Autodesk Inventor part; units mm, degrees
ref_plane "YZ Plane" through (0, 0, 0) normal (1, 0, 0) x (0, 1, 0)
ref_plane "XZ Plane" through (0, 0, 0) normal (0, 1, 0) x (-1, 0, 0)
ref_plane "XY Plane" through (0, 0, 0) normal (0, 0, 1) x (1, 0, 0)
sketch "Skizze1" plane through (0, 0, 0) normal (0, 0, 1) x (1, 0, 0)
  circle A0 centre (0, 0) radius 9.75
  dimension "d0" = 19.5
extrude "Extrusion1" add sketch "Skizze1" along normal blind 830
sketch "Skizze4" plane through (0, 0, 830) normal (0, 0, 1) x (1, 0, 0)
  arc A0 (0, -25) -> (0, 25) centre (0, 0) ccw
  line L0 (0, 0) -> (0, -25) construction
  line L1 (0, 0) -> (0, 27.5151) construction
  line L2 (0, 25) -> (-100, 25)
  line L3 (-100, 25) -> (-100, -25)
  line L4 (-100, -25) -> (0, -25)
  point P0 (0, 25)
  dimension "d9" = 180
  dimension "d10" = 100
  dimension "d11" = 50
  dimension "d12" = 25
extrude "Extrusion4" add sketch "Skizze4" along normal blind 10
sketch "Skizze5" plane through (0, 0, 0) normal (0, 0, -1) x (-1, 0, 0)
  arc A0 (0, 25) -> (0, -25) centre (0, 0) ccw
  line L0 (0, 25) -> (100, 25)
  line L1 (100, 25) -> (100, -25)
  line L2 (100, -25) -> (0, -25)
  dimension "d15" = 25
  dimension "d16" = 0
  dimension "d17" = 0
  dimension "d18" = 100
  dimension "d19" = 50
  dimension "d20" = 90
extrude "Extrusion5" add sketch "Skizze5" along normal blind 10
sketch "Skizze6" plane through (0, 0, 0) normal (0, 0, 1) x (1, 0, 0)
  circle A0 centre (-90, 0) radius 5
  line L0 (-100, 25) -> (0, 25)
  line L1 (-100, -25) -> (-100, 25)
  point P0 (0, 0)
  dimension "d23" = 10
  dimension "d24" = 25
  dimension "d25" = 10
extrude "Extrusion6" cut sketch "Skizze6" against normal up to surface (10 mm away)
sketch "Skizze7" plane through (0, 0, -10) normal (0, 0, -1) x (-1, 0, 0)
  circle A0 centre (0, 0) radius 9.75
  dimension "d28" = 19.5
extrude "Extrusion7" add sketch "Skizze7" along normal blind 15
sketch "Skizze8" plane through (0, 0, -25) normal (0, 0, -1) x (-1, 0, 0)
  line L0 (9.75, 0) -> (-9.75, 0)
  line L1 (-9.75, 0) -> (-9.75, 300)
  line L2 (-9.75, 300) -> (9.75, 300)
  line L3 (9.75, 300) -> (9.75, 0)
  circle A0 centre (0, 0) radius 9.75
  circle A1 centre (0, 0) radius 9.75
  dimension "d31" = 300
  dimension "d32" = 19.5
  dimension "d33" = 9.75
  dimension "d34" = 0
  dimension "d35" = 19.5
extrude "Extrusion8" add sketch "Skizze8" along normal blind 10
sketch "Skizze9" plane through (0, 0, -25) normal (0, 0, 1) x (1, 0, 0)
  circle A0 centre (0, 290) radius 6
  line L0 (9.75, 300) -> (9.75, 0)
  line L1 (-9.75, 300) -> (9.75, 300)
  point P0 (0, 0)
  dimension "d38" = 12
  dimension "d39" = 9.75
  dimension "d40" = 10
extrude "Extrusion9" cut sketch "Skizze9" against normal up to surface (10 mm away)
properties part number "LenkungHinten"
Read the model definition and answer for the solid it produces. Units are mm, in the model's axes. A direction names the side the tool comes from. Coordinates: 2 decimals unless noted, no trailing zeros. Loops run counter-clockwise (first coordinate to the right, second up) from the corner with the lowest first, then second, coordinate; pieces in that order, holes last. Notation, with made-up numbers: (-11.75, -36) -> (42.25, -36) arc R30 ccw to (42.25, 1) -> close; hole circle Ø5 at (-8.5, -39). An arc over 180 degrees is marked (long way). Answer in a Markdown table with one row per item.
Item 1: A cutting plane is placed at B-B on y = 85.5. Determine the outline of the cut face in (x, z), plus the area to 3 significant figures.
Returned:
| item | result |
|---|---|
| outline | (-9.75, -35) -> (9.75, -35) -> (9.75, -25) -> (-9.75, -25) -> close |
| area | 195 mm^2 |
Item 2: Straight lines are drawn through the part: line 1 along X through (y, z) = (290, -32.5); line 2 along Z through (x, y) = (-60, 15.5); line 3 along Y through (x, z) = (-90, -4.75). For each, find the intervals that lie inside material, in ascending order. Write a range as [from, to].
Returned:
| item | result |
|---|---|
| line 1 | x = [-9.75, -6], [6, 9.75] |
| line 2 | z = [-10, 0], [830, 840] |
| line 3 | y = [-25, -5], [5, 25] |
Item 3: For a pull along Z with two mould halves and no side action, classify faces 1 (the cylindrical face through (-1.269, -9.667, 409.19)), 2 (the flat face through (-38, 0, 840)), 3 (the cylindrical face through (24.994, 0.55, 834.93)), 4 (the flat face through (-37, 0, 0)) as released by +Z, released by -Z, zero draft, split by the parting line, or undercut.
Returned:
| item | result |
|---|---|
| face 1 | undercut |
| face 2 | released by +Z |
| face 3 | zero draft |
| face 4 | undercut |
Item 4: A cutting plane is placed at C-C on z = 327.5. Determine the outline of the cut face in (x, y).
Returned:
| item | result |
|---|---|
| outline | circle Ø19.5 at (0, 0) |
Item 5: Each of these flat-tipped pins is pushed along its axis until it touches: P1, Ø8, axis at x = -90, y = 0, coming from the -Z side; P2, Ø14, axis at x = 0, y = 290, coming from the +Z side; P3, Ø8, axis at x = -72, z = -5, coming from the +Y side. Where does it stop, or does it pass through?
Returned:
| item | result |
|---|---|
| P1 | stops at z = 830 |
| P2 | stops at z = -25 |
| P3 | stops at y = 25 |
Item 6: For faces 5 (the flat face through (0, 147, -35)), 6 (the cylindrical face through (1.269, -9.667, -19.547)), determine the directions among +Z, -Z, +X, -X, +Y, -Y from which every point of the face is accessible in a straight line to the end or side of a thin tool.
Returned:
| item | result |
|---|---|
| face 5 | -Z, +X, -X, +Y, -Y |
| face 6 | none |
Item 7: A cutting plane is placed at A-A on x = -20. Determine the outline of the cut face in (y, z), plus the area to 3 significant figures.
Returned:
| item | result |
|---|---|
| outline | (-25, -10) -> (25, -10) -> (25, 0) -> (-25, 0) -> close; (-25, 830) -> (25, 830) -> (25, 840) -> (-25, 840) -> close |
| area | 1,000 mm^2 |
